from build123d import *

# Parameters (mm, degrees)
SKETCH1_W           = 58.75
SKETCH1_H           = 49.25
SKETCH1_R           = 3.05
BOSS_EXTRUDE1_DEPTH = 1.5
BOSS_EXTRUDE2_DEPTH = 49.25
CUT_EXTRUDE1_DEPTH  = 2
CUT_EXTRUDE3_DEPTH  = 64.827526389
CHAMFER3_SIZE       = 2


with BuildPart() as part:
    # Sketch1 → Boss-Extrude1 (new body)
    with BuildSketch(Plane(origin=(0, 0, 0), x_dir=(1, 0, 0), z_dir=(0, 1, 0))):
        Rectangle(SKETCH1_W, SKETCH1_H)
        with Locations(Location((0, 0, 0), (0, 0, 270))):
            Circle(SKETCH1_R, mode=Mode.SUBTRACT)
    extrude(amount=BOSS_EXTRUDE1_DEPTH)

    # Sketch2 → Boss-Extrude2 (add)
    with BuildSketch(Plane(origin=(0, 0, -24.625), x_dir=(-1, 0, 0), z_dir=(0, 0, -1))):
        Polygon((-29.375, 1.5), (29.375, 1.5), (29.375, 2.5), (28.2, 4), (27.025, 2.5), (25.85, 4), (24.675, 2.5), (23.5, 4), (22.325, 2.5), (21.15, 4), (19.975, 2.5), (18.8, 4), (17.625, 2.5), (16.45, 4), (15.275, 2.5), (14.1, 4), (12.925, 2.5), (11.75, 4), (10.575, 2.5), (9.4, 4), (8.225, 2.5), (7.05, 4), (5.875, 2.5), (4.7, 4), (3.525, 2.5), (2.35, 4), (1.175, 2.5), (0, 4), (-1.175, 2.5), (-2.35, 4), (-3.525, 2.5), (-4.7, 4), (-5.875, 2.5), (-7.05, 4), (-8.225, 2.5), (-9.4, 4), (-10.575, 2.5), (-11.75, 4), (-12.925, 2.5), (-14.1, 4), (-15.275, 2.5), (-16.45, 4), (-17.625, 2.5), (-18.8, 4), (-19.975, 2.5), (-21.15, 4), (-22.325, 2.5), (-23.5, 4), (-24.675, 2.5), (-25.85, 4), (-27.025, 2.5), (-28.2, 4), (-29.375, 2.5), align=None)
    extrude(amount=-BOSS_EXTRUDE2_DEPTH)

    # Sketch3 → Cut-Extrude1 (cut)
    with BuildSketch(Plane(origin=(0, 0, 0), x_dir=(-1, 0, 0), z_dir=(0, -1, 0))):
        with BuildLine():
            Line((-1.75, -2.497999199), (-1.75, -5))
            Line((-1.75, -5), (1.75, -5))
            Line((1.75, -5), (1.75, -2.497999199))
            ThreePointArc((1.75, -2.497999199), (0, 3.05), (-1.75, -2.497999199))
        make_face()
    extrude(amount=-CUT_EXTRUDE1_DEPTH, mode=Mode.SUBTRACT)

    # Sketch4 → Cut-Extrude3 (cut, through all)
    with BuildSketch(Plane(origin=(29.375, 0, 0), x_dir=(0, 0, -1), z_dir=(1, 0, 0))):
        with BuildLine():
            Line((-23.875, 4), (-24.625, 4))
            Line((-24.625, 4), (-24.625, 3.25))
            ThreePointArc((-24.625, 3.25), (-24.405330086, 3.780330086), (-23.875, 4))
        make_face()
    cut_extrude3 = extrude(amount=-CUT_EXTRUDE3_DEPTH, mode=Mode.SUBTRACT)

    # Mirror1: Cut-Extrude3 across plane
    add(cut_extrude3.mirror(Plane.XY), mode=Mode.SUBTRACT)

    # Chamfer3
    chamfer3_edges = [part.edges().sort_by_distance(p)[0] for p in [
        (0, 0, 5),
    ]]
    chamfer(chamfer3_edges, length=CHAMFER3_SIZE - 0.0001)  # a hair under: the kernel refuses the full size


solid = part.part
Read the model definition and answer for the solid it produces. Units are mm, in the model's axes. A direction names the side the tool comes from. Give positions to 0.01 mm unless a question says otherwise; leave off trailing zeros. Answer in a Markdown table with one row per item. Add a question column.
Item 1: Flat-ended cylindrical pins translate along their axes: P1, Ø3.5, axis at x = 0, z = 0, coming from the -Y side; P2, Ø12, axis at x = -20, z = 4.5, coming from the +Y side. Find the tip coordinate at first contact, or state that the pin passes through.
Item 2: Determine the mould class of faces 1 (the face through (0, 0, -6)), 2 (the face through (-11.2, 3.3, -0.3)), 3 (the face through (9.98, 3.26, -0.34)) for opening direction X: pulls with the +X half, pulls with the -X half, needs draft (parallel to the pull), parting line crosses it, or undercut.
Item 3: Find the intervals of material crossed by L1, parallel to X at y = 1.65, z = 0 (3 decimals); L2, parallel to Z at x = 0, y = 1.7 (3 decimals); L3, parallel to Z at x = 0, y = 0.9 (3 decimals), in increasing order.
Item 4: A tool of negligible diameter and unlimited length cuts with its end or side. For faces 4 (the face through (-1.75, 1, 4)), 5 (the face through (-21.746, 3.24, -0.345)), from which of +Z, -Z, +X, -X, +Y, -Y can it reach the whole face along a straight path? Write none if from no direction.
Recorded:
| question | item | result |
|---|---|---|
| 1 | P1 | stops at y = 2 |
| 1 | P2 | stops at y = 4 |
| 2 | face 1 | needs draft |
| 2 | face 2 | undercut |
| 2 | face 3 | undercut |
| 3 | L1 | x = -29.375 to -3.05, 3.05 to 29.375 |
| 3 | L2 | z = -24.625 to -3.05, 5.3 to 24.625 |
| 3 | L3 | z = -24.625 to -3.05, 6.1 to 24.625 |
| 4 | face 4 | -Y |
| 4 | face 5 | +Z, -Z, +Y |
